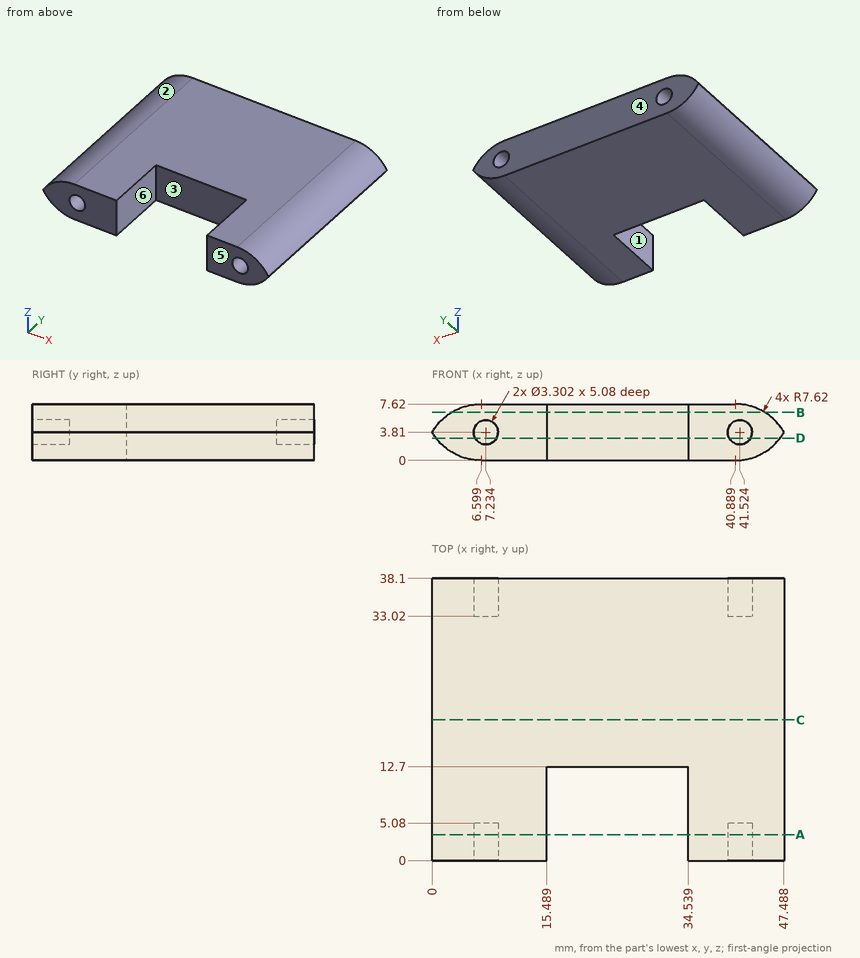
Could you check a few things on this drawing? It's one solid part, dimensions in mm from its lowest x, y, z. A direction names the side the tool comes from. Coordinates: 2 decimals unless noted, no trailing zeros. Order: outer loops, then holes, each group sorted by start corner. A loop starts at its lowest first (then second) coordinate and runs counter-clockwise, first axis right, second up. Notation, with made-up numbers: M 84.5,89.25 L 112.5,89.25 A30 cw 112.5,114.25 Z; hole C 48,4.5 d4. An arc over 180 degrees is marked long. Use a Markdown table: item, result. Add a question column.
Q1. Which directions (+Z, -Z, +X, -X, +Y, -Y) give clear straight access to the entire face, cutting with the end or side of a thin tool? Please do the marked faces 5 and 6.
Q2. I want a section at C-C on y = 19. List the corners of the cut face in (x, z) for me.
Q3. I'm going to push flat-ended pins straight in: pin 1 (1 mm diameter, centred on x = 7, z = 3, fed in from -Y); pin 2 (3.5 mm diameter, centred on x = 41, z = 3.5, fed in from +Y); pin 3 (2.5 mm diameter, centred on y = 3, z = 2.5, fed in from +X); pin 4 (1.5 mm diameter, centred on x = 28.5, y = 11.5, fed in from +Z). Where does each tip first touch, or does it pass through?
Q4. I want a section at D-D on z = 3. List the corners of the cut face in (x, y) for me, then the cut area to 3 significant figures.
Q5. I want a section at A-A on y = 3.5. List the corners of the cut face in (x, z) for me.
Q6. I want a section at B-B on z = 6.5. List the corners of the cut face in (x, y) for me.
Q7. We'd pull the mould along X, two halves only. Please class the marked faces 1, 2, 3 and 4: pulls with the +X half, pulls with the -X half, needs draft (parallel to the pull), parting line crosses it, or undercut.
Q8. If I drill on L1, parallel to X at y = 2.95, z = 3.81 (1 decimal); L2, parallel to X at y = 35.6, z = 3.81 (1 decimal); L3, parallel to Y at x = 31, z = 6, over which ranges is the centre line in solid material (lowest first)?
Checked values:
| question | item | result |
|---|---|---|
| 1 | face 5 | +Z, -Z, +X, -X, -Y |
| 1 | face 6 | +Z, -Z, -Y |
| 2 | outline | M 0,3.81 A7.62 ccw 6.6,0 L 40.89,0 A7.62 ccw 47.49,3.81 A7.62 ccw 40.89,7.62 L 6.6,7.62 A7.62 ccw Z |
| 3 | pin 1 | y = 5.08 |
| 3 | pin 2 | y = 38.1 |
| 3 | pin 3 | x = 47.45 |
| 3 | pin 4 | through |
| 4 | outline | M 0.54,0 L 5.8,0 L 5.8,5.08 L 8.67,5.08 L 8.67,0 L 15.49,0 L 15.49,12.7 L 34.54,12.7 L 34.54,0 L 40.09,0 L 40.09,5.08 L 42.96,5.08 L 42.96,0 L 46.95,0 L 46.95,38.1 L 42.96,38.1 L 42.96,33.02 L 40.09,33.02 L 40.09,38.1 L 8.67,38.1 L 8.67,33.02 L 5.8,33.02 L 5.8,38.1 L 0.54,38.1 Z |
| 4 | area | 1,470 mm² |
| 5 | outline | M 0,3.81 A7.62 ccw 6.6,0 L 15.49,0 L 15.49,7.62 L 6.6,7.62 A7.62 ccw Z; M 34.54,0 L 40.89,0 A7.62 ccw 47.49,3.81 A7.62 ccw 40.89,7.62 L 34.54,7.62 Z; hole C 7.23,3.81 d3.3; hole C 41.52,3.81 d3.3 |
| 6 | outline | M 2.62,0 L 15.49,0 L 15.49,12.7 L 34.54,12.7 L 34.54,0 L 44.87,0 L 44.87,38.1 L 2.62,38.1 Z |
| 7 | face 1 | undercut |
| 7 | face 2 | pulls with the -X half |
| 7 | face 3 | undercut |
| 7 | face 4 | needs draft |
| 8 | L1 | 0 to 5.6, 8.9 to 15.5, 34.5 to 39.9, 43.2 to 47.5 |
| 8 | L2 | 0 to 5.6, 8.9 to 39.9, 43.2 to 47.5 |
| 8 | L3 | 12.7 to 38.1 |
